Geometry: see drawing. Coordinates: mm, zero at the bounding-box minimum. A direction names the side the tool comes from. Give positions to 0.01 mm unless a question says otherwise; leave off trailing zeros. Loops run counter-clockwise (first coordinate to the right, second up) from the corner with the lowest first, then second, coordinate; pieces in that order, holes last. Notation, with made-up numbers: (42, 71.5) - (64, 71.5) arc R21 cw to (64, 99.5) - close; hole circle Ø11 at (-15.5, 9.25). An arc over 180 degrees is marked (long way). Use one line per item in the form item = value.
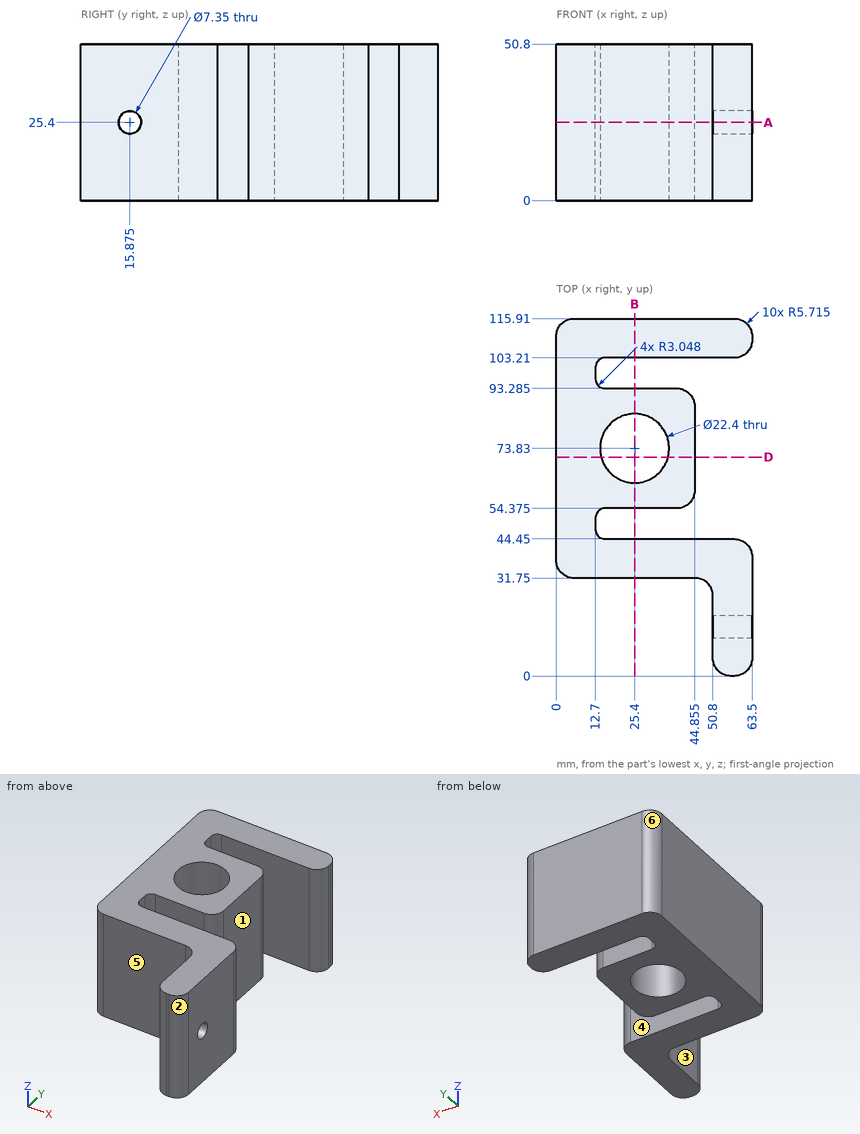
(1) Pin query (flat end, axial travel): P1, Ø13.5, axis at y = 73, z = 16, coming from the +X side (3 decimals); P2, Ø9.5, axis at y = 15.875, z = 25.4, coming from the -X side; P3, Ø12.5, axis at x = 40, z = 37.5, coming from the -Y side; P4, Ø5, axis at x = 27.5, y = 99.5, coming from the +Z side. Return the tip coordinate at first contact, or that it passes through.
Solution:
P1 = 44.855
P2 = 50.8
P3 = 31.63
P4 = through
(2) Pull-direction query (Y, two-part tool) for the marked faces 4, 5 and 6; classes: released by +Y, released by -Y, zero draft, split by the parting line, or undercut.
Solution:
face_4 = undercut
face_5 = released by -Y
face_6 = released by +Y
(3) Material intervals for L1, parallel to Y at x = 25, z = 16 (3 decimals); L2, parallel to Y at x = 57.5, z = 48; L3, parallel to Y at x = 23, z = 41 (3 decimals), sorted ascending. Write a range as from..to.
Solution:
L1 = 31.75..44.45, 54.375..62.637, 85.023..93.285, 103.21..115.91
L2 = 0..44.45, 103.21..115.91
L3 = 31.75..44.45, 54.375..62.89, 84.77..93.285, 103.21..115.91
(4) Cut plane B-B (x = 25.4). Return the cut outline in (y, z) (3 decimals), plus the area to 3 significant figures.
Solution:
outline = (31.75, 0) - (44.45, 0) - (44.45, 50.8) - (31.75, 50.8) - close; (54.375, 0) - (62.63, 0) - (62.63, 50.8) - (54.375, 50.8) - close; (85.03, 0) - (93.285, 0) - (93.285, 50.8) - (85.03, 50.8) - close; (103.21, 0) - (115.91, 0) - (115.91, 50.8) - (103.21, 50.8) - close
area = 2,130 mm2
(5) Cut plane A-A (z = 25.4). Give the number of separate pieces and of enclosed holes in the cut face, plus the area to 3 significant figures.
Solution:
separate_pieces = 2
enclosed_holes = 1
area = 3,480 mm2
(6) Access query for the marked faces 1, 2 and 3. Directions: +Z, -Z, +X, -X, +Y, -Y. A direction counts if a zero-diameter tool reaches every point of the face in a straight line with its end or side. Return the directions, or none.
Solution:
face_1 = +Z, -Z, +X
face_2 = +Z, -Z, +X, -Y
face_3 = +Z, -Z, -X, -Y
(7) Cut plane D-D (y = 71). Return the cut outline in (x, z) (3 decimals), plus the area to 3 significant figures.
Solution:
outline = (0, 0) - (14.563, 0) - (14.563, 50.8) - (0, 50.8) - close; (36.237, 0) - (44.855, 0) - (44.855, 50.8) - (36.237, 50.8) - close
area = 1,180 mm2
